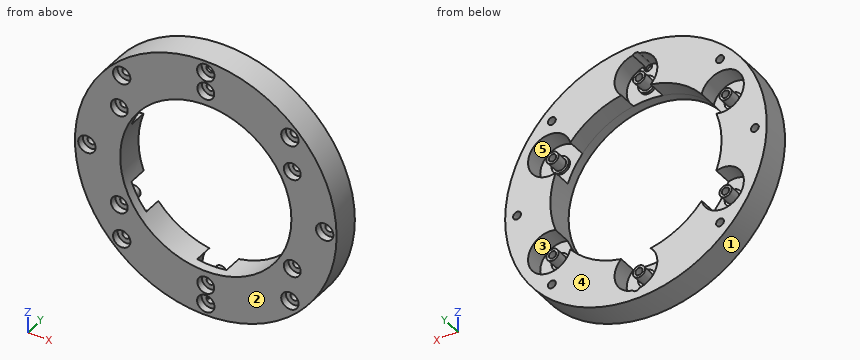
from build123d import *

# Parameters (mm, degrees)
SKETCH1_R           = 55
SKETCH1_R_2         = 36
SKETCH1_R_3         = 1.55
BOSS_EXTRUDE1_DEPTH = 4
SKETCH3_R           = 3.55
SKETCH3_R_2         = 1.55
BOSS_EXTRUDE2_DEPTH = 1
SKETCH5_R           = 2.55
SKETCH5_R_2         = 1.55
BOSS_EXTRUDE3_DEPTH = 5
SKETCH6_R           = 55
BOSS_EXTRUDE4_DEPTH = 8
SKETCH8_R           = 1.65
CUT_EXTRUDE2_DEPTH  = 13
SKETCH7_R           = 3.55
SKETCH7_R_2         = 1.55
SKETCH7_R_3         = 3.65
SKETCH7_R_4         = 1.65
CUT_EXTRUDE1_DEPTH  = 3


with BuildPart() as part:
    # Sketch1 → Boss-Extrude1 (new body)
    with BuildSketch(Plane(origin=(0, 0, 0), x_dir=(1, 0, 0), z_dir=(0, 1, 0))):
        Circle(SKETCH1_R)
        Circle(SKETCH1_R_2, mode=Mode.SUBTRACT)
        with Locations((0, 42)):
            Circle(SKETCH1_R_3, mode=Mode.SUBTRACT)
        with Locations((36.373066959, 21)):
            Circle(SKETCH1_R_3, mode=Mode.SUBTRACT)
        with Locations((36.373066959, -21)):
            Circle(SKETCH1_R_3, mode=Mode.SUBTRACT)
        with Locations((0, -42)):
            Circle(SKETCH1_R_3, mode=Mode.SUBTRACT)
        with Locations((-36.373066959, -21)):
            Circle(SKETCH1_R_3, mode=Mode.SUBTRACT)
        with Locations((-36.373066959, 21)):
            Circle(SKETCH1_R_3, mode=Mode.SUBTRACT)
    extrude(amount=BOSS_EXTRUDE1_DEPTH)

    # Sketch3 → Boss-Extrude2 (add)
    with BuildSketch(Plane(origin=(0, 4, 0), x_dir=(1, 0, 0), z_dir=(0, 1, 0))):
        with Locations((-36.373066959, 21)):
            Circle(SKETCH3_R)
        with Locations((-36.373066959, 21)):
            Circle(SKETCH3_R_2, mode=Mode.SUBTRACT)
        with Locations((0, -42)):
            Circle(SKETCH3_R)
        with Locations((0, -42)):
            Circle(SKETCH3_R_2, mode=Mode.SUBTRACT)
        with Locations((36.373066959, 21)):
            Circle(SKETCH3_R)
        with Locations((36.373066959, 21)):
            Circle(SKETCH3_R_2, mode=Mode.SUBTRACT)
        with Locations((0, 42)):
            Circle(SKETCH3_R)
        with Locations((0, 42)):
            Circle(SKETCH3_R_2, mode=Mode.SUBTRACT)
        with Locations((36.373066959, -21)):
            Circle(SKETCH3_R)
        with Locations((36.373066959, -21)):
            Circle(SKETCH3_R_2, mode=Mode.SUBTRACT)
        with Locations((-36.373066959, -21)):
            Circle(SKETCH3_R)
        with Locations((-36.373066959, -21)):
            Circle(SKETCH3_R_2, mode=Mode.SUBTRACT)
    extrude(amount=BOSS_EXTRUDE2_DEPTH)

    # Sketch5 → Boss-Extrude3 (add)
    with BuildSketch(Plane(origin=(0, 5, 0), x_dir=(1, 0, 0), z_dir=(0, 1, 0))):
        with Locations((-36.373066959, -21)):
            Circle(SKETCH5_R)
        with Locations((-36.373066959, -21)):
            Circle(SKETCH5_R_2, mode=Mode.SUBTRACT)
        with Locations((0, -42)):
            Circle(SKETCH5_R)
        with Locations((0, -42)):
            Circle(SKETCH5_R_2, mode=Mode.SUBTRACT)
        with Locations((36.373066959, -21)):
            Circle(SKETCH5_R)
        with Locations((36.373066959, -21)):
            Circle(SKETCH5_R_2, mode=Mode.SUBTRACT)
        with Locations((36.373066959, 21)):
            Circle(SKETCH5_R)
        with Locations((36.373066959, 21)):
            Circle(SKETCH5_R_2, mode=Mode.SUBTRACT)
        with Locations((0, 42)):
            Circle(SKETCH5_R)
        with Locations((0, 42)):
            Circle(SKETCH5_R_2, mode=Mode.SUBTRACT)
        with Locations((-36.373066959, 21)):
            Circle(SKETCH5_R)
        with Locations((-36.373066959, 21)):
            Circle(SKETCH5_R_2, mode=Mode.SUBTRACT)
    extrude(amount=BOSS_EXTRUDE3_DEPTH)

    # Sketch6 → Boss-Extrude4 (add)
    with BuildSketch(Plane(origin=(0, 4, 0), x_dir=(1, 0, 0), z_dir=(0, 1, 0))):
        Circle(SKETCH6_R)
        with BuildLine():
            ThreePointArc((6.187442022, 35.464285714), (0, 51), (-6.187442022, 35.464285714))
            ThreePointArc((-6.187442022, 35.464285714), (-18, 31.176914536), (-27.619251345, 23.090624833))
            ThreePointArc((-27.619251345, 23.090624833), (-44.167295593, 25.5), (-33.806693367, 12.373660882))
            ThreePointArc((-33.806693367, 12.373660882), (-36, 0), (-33.806693367, -12.373660882))
            ThreePointArc((-33.806693367, -12.373660882), (-44.167295593, -25.5), (-27.619251345, -23.090624833))
            ThreePointArc((-27.619251345, -23.090624833), (-18, -31.176914536), (-6.187442022, -35.464285714))
            ThreePointArc((-6.187442022, -35.464285714), (0, -51), (6.187442022, -35.464285714))
            ThreePointArc((6.187442022, -35.464285714), (18, -31.176914536), (27.619251345, -23.090624833))
            ThreePointArc((27.619251345, -23.090624833), (44.167295593, -25.5), (33.806693367, -12.373660882))
            ThreePointArc((33.806693367, -12.373660882), (36, 0), (33.806693367, 12.373660882))
            ThreePointArc((33.806693367, 12.373660882), (44.167295593, 25.5), (27.619251345, 23.090624833))
            ThreePointArc((27.619251345, 23.090624833), (18, 31.176914536), (6.187442022, 35.464285714))
        make_face(mode=Mode.SUBTRACT)
    extrude(amount=BOSS_EXTRUDE4_DEPTH)

    # Sketch8 → Cut-Extrude2 (cut, through all)
    with BuildSketch(Plane(origin=(0, 12, 0), x_dir=(1, 0, 0), z_dir=(0, 1, 0))):
        with Locations((0, 50)):
            Circle(SKETCH8_R)
        with Locations((35.355339059, 35.355339059)):
            Circle(SKETCH8_R)
        with Locations((50, 0)):
            Circle(SKETCH8_R)
        with Locations((35.355339059, -35.355339059)):
            Circle(SKETCH8_R)
        with Locations((0, -50)):
            Circle(SKETCH8_R)
        with Locations((-35.355339059, -35.355339059)):
            Circle(SKETCH8_R)
        with Locations((-50, 0)):
            Circle(SKETCH8_R)
        with Locations((-35.355339059, 35.355339059)):
            Circle(SKETCH8_R)
    extrude(amount=-CUT_EXTRUDE2_DEPTH, mode=Mode.SUBTRACT)

    # Sketch7 → Cut-Extrude1 (cut)
    with BuildSketch(Plane.XZ):
        with Locations((-36.373066959, -21)):
            Circle(SKETCH7_R)
        with Locations((-36.373066959, -21)):
            Circle(SKETCH7_R_2, mode=Mode.SUBTRACT)
        with Locations((-36.373066959, 21)):
            Circle(SKETCH7_R)
        with Locations((-36.373066959, 21)):
            Circle(SKETCH7_R_2, mode=Mode.SUBTRACT)
        with Locations((0, 42)):
            Circle(SKETCH7_R)
        with Locations((0, 42)):
            Circle(SKETCH7_R_2, mode=Mode.SUBTRACT)
        with Locations((36.373066959, 21)):
            Circle(SKETCH7_R)
        with Locations((36.373066959, 21)):
            Circle(SKETCH7_R_2, mode=Mode.SUBTRACT)
        with Locations((36.373066959, -21)):
            Circle(SKETCH7_R)
        with Locations((36.373066959, -21)):
            Circle(SKETCH7_R_2, mode=Mode.SUBTRACT)
        with Locations((0, -42)):
            Circle(SKETCH7_R)
        with Locations((0, -42)):
            Circle(SKETCH7_R_2, mode=Mode.SUBTRACT)
        with Locations((-35.355339059, -35.355339059)):
            Circle(SKETCH7_R_3)
        with Locations((-35.355339059, -35.355339059)):
            Circle(SKETCH7_R_4, mode=Mode.SUBTRACT)
        with Locations((-50, 0)):
            Circle(SKETCH7_R_3)
        with Locations((-50, 0)):
            Circle(SKETCH7_R_4, mode=Mode.SUBTRACT)
        with Locations((-35.355339059, 35.355339059)):
            Circle(SKETCH7_R_3)
        with Locations((-35.355339059, 35.355339059)):
            Circle(SKETCH7_R_4, mode=Mode.SUBTRACT)
        with Locations((0, 50)):
            Circle(SKETCH7_R_3)
        with Locations((0, 50)):
            Circle(SKETCH7_R_4, mode=Mode.SUBTRACT)
        with Locations((35.355339059, 35.355339059)):
            Circle(SKETCH7_R_3)
        with Locations((35.355339059, 35.355339059)):
            Circle(SKETCH7_R_4, mode=Mode.SUBTRACT)
        with Locations((50, 0)):
            Circle(SKETCH7_R_3)
        with Locations((50, 0)):
            Circle(SKETCH7_R_4, mode=Mode.SUBTRACT)
        with Locations((35.355339059, -35.355339059)):
            Circle(SKETCH7_R_3)
        with Locations((35.355339059, -35.355339059)):
            Circle(SKETCH7_R_4, mode=Mode.SUBTRACT)
        with Locations((0, -50)):
            Circle(SKETCH7_R_3)
        with Locations((0, -50)):
            Circle(SKETCH7_R_4, mode=Mode.SUBTRACT)
    extrude(amount=-CUT_EXTRUDE1_DEPTH, mode=Mode.SUBTRACT)


solid = part.part
For this review, take the finished solid that the model builds, in its own axes (mm). Face numbers are marked on the shaded views. A direction names the side the tool comes from. Give positions to 0.01 mm unless a question says otherwise; leave off trailing zeros. Loops run counter-clockwise (first coordinate to the right, second up) from the corner with the lowest first, then second, coordinate; pieces in that order, holes last. Notation, with made-up numbers: M -0.5,-23.5 L 18.5,-23.5 A21 ccw 18.5,10.5 Z; hole C 75.25,1 d5. An arc over 180 degrees is marked long. Put each result on its own line as item: value. Start each with the question number.
(1) Add section A-A, the plane z = 42. Write out the cut boundary in (x, y), then the cut area to 3 significant figures.
(2) For pin 1 (1 mm diameter, centred on y = 9.5, z = -19, fed in from -X); pin 2 (4 mm diameter, centred on x = -37, z = 22, fed in from +Y); pin 3 (2 mm diameter, centred on x = -37, z = 20, fed in from -Y), all flat-tipped, find the tip position at first contact; note any pin that passes through.
(3) Add section D-D, the plane z = -8.5. Write out the cut boundary in (x, y).
(4) Wall thickness on L1, parallel to X at y = 8.5, z = 0; L2, parallel to Z at x = 0, y = 1.2; L3, parallel to Z at x = -43, y = 6.75: over which ranges is each line inside the solid? List them lowest first.
(5) Add section B-B, the plane x = 0. Give the number of separate pieces and of enclosed holes in the cut face, then the cut area to 3 significant figures.
(6) Machinability: for the marked faces 4 and 5, which of the approach directions +Z, -Z, +X, -X, +Y, -Y give a long, thin tool a straight path to every point of the face, cutting with its end or side? Answer none if there is none.
(7) The part is to be moulded in two halves that separate along Z. For the marked faces 1, 2 and 3, say which applies: +Z half, -Z half, draft (parallel to the pull), parting line (faces both ways), or undercut.
Result:
1. outline: M -35.51,0 L -3.55,0 L -3.55,3 L -1.55,3 L -1.55,10 L -2.55,10 L -2.55,5 L -3.55,5 L -3.55,4 L -9,4 L -9,12 L -35.51,12 Z; M 1.55,3 L 3.55,3 L 3.55,0 L 35.51,0 L 35.51,12 L 9,12 L 9,4 L 3.55,4 L 3.55,5 L 2.55,5 L 2.55,10 L 1.55,10 Z
1. area: 698 mm^2
2. pin 1: stops at x = -51.8
2. pin 2: stops at y = 10
2. pin 3: stops at y = 3
3. outline: M -54.34,0 L -34.98,0 L -34.98,12 L -54.34,12 Z; M 34.98,0 L 54.34,0 L 54.34,12 L 34.98,12 Z
4. L1: x = -55 to -51.65, -48.35 to -36, 36 to 48.35, 51.65 to 55
4. L2: z = -55 to -53.65, -46.35 to -45.55, -38.45 to -36, 36 to 38.45, 45.55 to 46.35, 53.65 to 55
4. L3: z = -34.29 to -27.09, -14.91 to 14.91, 27.09 to 34.29
5. separate pieces: 6
5. enclosed holes: 0
5. area: 134 mm^2
6. face 4: +Z, -Z, +X, -X, +Y
6. face 5: +Y
7. face 1: parting line
7. face 2: draft
7. face 3: undercut
